Build history of the part. All positions in model axes, mm. A direction names the side the tool comes from. Give positions to 0.01 mm unless a question says otherwise; leave off trailing zeros. Write each loop counter-clockwise with the first axis right and the second up, starting at its lowest first coordinate (ties: lowest second). Pieces come first, ordered by that corner, then holes. Notation, with made-up numbers: (87.5, 23) -> (103.5, 23) arc R20 cw to (103.5, 50) -> close; hole circle Ø11 at (46.25, -39). An arc over 180 degrees is marked (long way). Put each result on its own line as item: value. Start each with the question number.
Item 1: Two-plate mould, pull along Y, no slides. Class faces 3 (the flat face through (14, 3.3, 123)), 4 (the flat face through (12, 0, 123)), 5 (the flat face through (9, 3, 249.043)), 6 (the cylindrical face through (1.67, 12.77, 127.32)): pulls with the +Y half, pulls with the -Y half, needs draft (parallel to the pull), parting line crosses it, or undercut.
Item 2: Slice it at C-C, the plane z = 202. List the corners of the cut face in (x, y).
Item 3: Flat gauge pins, fed straight in: pin 1 Ø8 at (x, z) = (8, 192.5) entering from +Y; pin 2 Ø2 at (y, z) = (11.5, 30) entering from +X. Where does each tip first touch, or does it go through?
Item 4: Slice it at A-A, the plane x = 18.8. List the corners of the cut face in (y, z), plus the area to 3 significant figures.
Item 5: Drill centre lines: line 1 along Z through (x, y) = (18.8, 0.9); line 2 along X through (y, z) = (17.5, 199). Where is each one in solid material? Low to high.
Item 6: Slice it at B-B, the plane y = 12.65. List the corners of the cut face in (x, z).
Item 7: Tool access for faces 1 (the flat face through (3.3, 16, 123)), 2 (the cylindrical face through (1.67, 19.18, 237.56)): list every direction of +Z, -Z, +X, -X, +Y, -Y with a clear straight run to the whole face (end or side of a thin tool).
Autodesk Inventor part; units mm, degrees
ref_plane "YZ Plane" through (0, 0, 0) normal (1, 0, 0) x (0, 1, 0)
ref_plane "XZ Plane" through (0, 0, 0) normal (0, 1, 0) x (-1, 0, 0)
ref_plane "XY Plane" through (0, 0, 0) normal (0, 0, 1) x (1, 0, 0)
sketch "Sketch1" plane through (0, 0, 0) normal (0, 0, 1) x (1, 0, 0)
  line L0 (0.5, 0) -> (3.3, 0)
  line L1 (3.3, 3.8) -> (3.3, 24.8)
  line L2 (2.8, 25.3) -> (0.5, 25.3)
  line L3 (0, 24.8) -> (0, 0.5)
  line L4 (0, 0) -> (24.8, 0)
  line L5 (25.3, 0.5) -> (25.3, 2.8)
  line L6 (24.8, 3.3) -> (3.8, 3.3)
  line L7 (0, 3.3) -> (0, 0)
  arc A0 (3.3, 24.8) -> (2.8, 25.3) centre (2.8, 24.8) ccw
  arc A1 (0.5, 25.3) -> (0, 24.8) centre (0.5, 24.8) ccw
  arc A2 (3.3, 3.8) -> (3.8, 3.3) centre (3.8, 3.8) ccw
  arc A3 (0, 0.5) -> (0.5, 0) centre (0.5, 0.5) ccw
  arc A4 (24.8, 0) -> (25.3, 0.5) centre (24.8, 0.5) ccw
  arc A5 (25.3, 2.8) -> (24.8, 3.3) centre (24.8, 2.8) ccw
  point P0 (3.3, 25.3)
  point P1 (0, 25.3)
  point P2 (25.3, 3.3)
  point P3 (25.3, 0)
  dimension "d0" = 3.3
  dimension "d1" = 25.3
  dimension "d2" = 25.3
  dimension "d3" = 3.3
  dimension "d4" = 0.5
extrude "Extrusion1" add sketch "Sketch1" along normal blind 249.043 contours A3 L3 A1 L2 A0 L1 A2 L6 A5 L5 A4 L4 L0
sketch "Sketch2" plane through (3.8, 3.3, 0) normal (0, 1, 0) x (1, 0, 0)
  circle A0 centre (15, -231.1777) radius 3.3
  line L0 (21, -249.043) -> (0, -249.043)
  line L1 (-3.8, 0) -> (-3.8, -249.043) construction
  line L2 (-3.8, -124.5215) -> (21, -124.5215) construction
  line L3 (21, 0) -> (21, -249.043) construction
  circle A1 centre (15, -17.8653) radius 3.3
  line L4 (15, -231.1777) -> (15, -124.5215) construction
  line L5 (15, -124.5215) -> (15, -17.8653) construction
  circle A2 centre (15, -75.1918) radius 3.3
  circle A3 centre (15, -173.8512) radius 3.3
  dimension "d7" = 6.6
  dimension "d9" = 6
  dimension "d12" = 213.3123
  dimension "d23" = 6.6
extrude "Extrusion2" cut sketch "Sketch2" against normal through all
sketch "Sketch3" plane through (3.3, 3.8, 0) normal (1, 0, 0) x (0, 0, -1)
  line L0 (-249.043, 21) -> (-249.043, -3.3) construction
  line L1 (-249.043, 8.85) -> (0, 8.85) construction
  line L2 (0, 21) -> (0, -3.3)
  circle A0 centre (-124.5215, 8.85) radius 2.8
  circle A1 centre (-207.5358, 8.85) radius 2.8
  circle A2 centre (-41.5072, 8.85) radius 2.8
  line L3 (-249.043, 0) -> (-249.043, 21)
  line L4 (0, 21.5) -> (-249.043, 21.5)
  line L5 (-249.043, 21.5) -> (-249.043, 21)
  arc A3 (-262.8543, 11.011) -> (-243.3985, 118.5449) centre (-259.3098, 65.8967) ccw
  point P0 (0, -3.8)
  point P1 (-249.043, 11.8634)
  point P2 (-226.8454, 21.5)
  dimension "d14" = 5.6
  dimension "d15" = 249.043
  dimension "d16" = 124.5215
  dimension "d17" = 5.6
  dimension "d18" = 5.6
  dimension "d19" = 41.5072
  dimension "d20" = 41.5072
extrude "Extrusion3" cut sketch "Sketch3" against normal blind 10
equation "\"d16\" = 0.5 * d15"
equation "\"d19\" = 0.333333 * d16"
equation "\"d20\" = 0.333333 * d16"
properties part number "1in Angle x 250" material "Aluminum 6061"
Values follow:
1. face 3: pulls with the +Y half
1. face 4: pulls with the -Y half
1. face 5: needs draft
1. face 6: undercut
2. outline: (0, 0.5) arc R0.5 ccw to (0.5, 0) -> (24.8, 0) arc R0.5 ccw to (25.3, 0.5) -> (25.3, 2.8) arc R0.5 ccw to (24.8, 3.3) -> (3.8, 3.3) arc R0.5 cw to (3.3, 3.8) -> (3.3, 24.8) arc R0.5 ccw to (2.8, 25.3) -> (0.5, 25.3) arc R0.5 ccw to (0, 24.8) -> close
3. pin 1: y = 3.3
3. pin 2: x = 3.3
4. outline: (0, 0) -> (3.3, 0) -> (3.3, 14.57) -> (0, 14.57) -> close; (0, 21.17) -> (3.3, 21.17) -> (3.3, 71.89) -> (0, 71.89) -> close; (0, 78.49) -> (3.3, 78.49) -> (3.3, 170.55) -> (0, 170.55) -> close; (0, 177.15) -> (3.3, 177.15) -> (3.3, 227.88) -> (0, 227.88) -> close; (0, 234.48) -> (3.3, 234.48) -> (3.3, 249.04) -> (0, 249.04) -> close
4. area: 735 mm2
5. line 1: 0 to 14.57, 21.17 to 71.89, 78.49 to 170.55, 177.15 to 227.88, 234.48 to 249.04
5. line 2: 0 to 3.3
6. outline: (0, 0) -> (3.3, 0) -> (3.3, 38.71) -> (0, 38.71) -> close; (0, 44.31) -> (3.3, 44.31) -> (3.3, 121.72) -> (0, 121.72) -> close; (0, 127.32) -> (3.3, 127.32) -> (3.3, 204.74) -> (0, 204.74) -> close; (0, 210.34) -> (3.3, 210.34) -> (3.3, 249.04) -> (0, 249.04) -> close
7. face 1: +Z, -Z, +X, +Y
7. face 2: +Z, +X, -X, +Y
